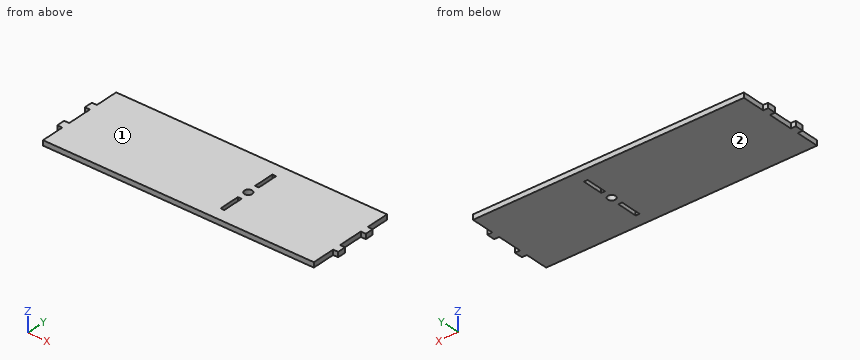
from build123d import *

# Parameters (mm, degrees)
SKETCH1_W           = 1.8
SKETCH1_H           = 10
SKETCH1_R           = 1.9
BOSS_EXTRUDE1_DEPTH = 2.4


with BuildPart() as part:
    # Sketch1 → Boss-Extrude1 (new body)
    with BuildSketch(Plane.XY):
        Polygon((65, 21.15), (-65, 21.15), (-65, 10), (-67.4, 10), (-67.4, 6), (-65, 6), (-65, -6), (-67.4, -6), (-67.4, -10), (-65, -10), (-65, -21.15), (65, -21.15), (65, -10), (67.4, -10), (67.4, -6), (65, -6), (65, 6), (67.4, 6), (67.4, 10), (65, 10), align=None)
        with Locations((16, -10)):
            Rectangle(SKETCH1_W, SKETCH1_H, mode=Mode.SUBTRACT)
        with Locations((16, 0)):
            Circle(SKETCH1_R, mode=Mode.SUBTRACT)
        Polygon((16.9, 5), (16, 5), (15.1, 5), (15.1, 15), (16.9, 15), align=None, mode=Mode.SUBTRACT)
    extrude(amount=BOSS_EXTRUDE1_DEPTH)


solid = part.part
Geometry: final body of the model. Coordinates: model frame, mm. Face numbers are marked on the shaded views. Give positions to 0.01 mm unless a question says otherwise; leave off trailing zeros. Write each loop counter-clockwise with the first axis right and the second up, starting at its lowest first coordinate (ties: lowest second). Pieces come first, ordered by that corner, then holes.
(1) Cut plane A-A, the plane y = 0. Return loops of the section in (x, z), then the cut area to 3 significant figures.
(2) Ray query, line 1 (Y direction, x = 16, z = 0.85); line 2 (X direction, y = 8.5, z = 1.7); line 3 (Y direction, x = 15, z = 1.5). Return the intervals inside material, ascending.
(3) Cut plane B-B, the plane z = 2. Give the number of separate pieces and of enclosed holes in the cut face, then the cut area to 3 significant figures.
(4) First-contact query: P1, Ø2.5, axis at x = 16, y = 0, coming from the +Z side; P2, Ø4, axis at x = 28, y = -0.5, coming from the -Z side; P3, Ø1.2, axis at x = 66.5, z = 1, coming from the +Y side; P4, Ø0.7, axis at y = -14.5, z = 1, coming from the +X side. Flat tips, straight axial feed; report the tip coordinate or a pass-through.
(5) Cut plane C-C, the plane y = -17.5. Return loops of the section in (x, z), then the cut area to 3 significant figures.
(6) Mould query, pull axis Z, two halves, no side actions, for the marked faces 1 and 2. Classes: released by +Z, released by -Z, zero draft, split by the parting line, or undercut.
Values follow:
1. outline: (-65, 0) - (14.1, 0) - (14.1, 2.4) - (-65, 2.4) - close; (17.9, 0) - (65, 0) - (65, 2.4) - (17.9, 2.4) - close
1. area: 303 mm2
2. line 1: y = -21.15 to -15, -5 to -1.9, 1.9 to 5, 15 to 21.15
2. line 2: x = -67.4 to 15.1, 16.9 to 67.4
2. line 3: y = -21.15 to -1.62, 1.62 to 21.15
3. separate pieces: 1
3. enclosed holes: 3
3. area: 5,490 mm2
4. P1: passes through
4. P2: stops at z = 0
4. P3: stops at y = 10
4. P4: stops at x = 65
5. outline: (-65, 0) - (65, 0) - (65, 2.4) - (-65, 2.4) - close
5. area: 312 mm2
6. face 1: released by +Z
6. face 2: released by -Z
